Can you work these out from the model? Positions are in its coordinate system, mm. Face numbers are marked on the shaded views. A direction names the side the tool comes from. Give positions to 0.01 mm unless a question says otherwise; leave off trailing zeros. Write each loop counter-clockwise with the first axis right and the second up, starting at its lowest first coordinate (ties: lowest second). Pieces come first, ordered by that corner, then holes.
Autodesk Fusion 360 part; units mm, degrees
sketch "Boceto1" plane through (0, 0, 0) normal (0, 0, 1) x (1, 0, 0)
  line L0 (0, 0) -> (47.682, 0)
  line L1 (47.682, 0) -> (47.682, 36)
  line L2 (47.682, 36) -> (0, 36)
  line L3 (0, 36) -> (0, 0)
  line L4 (4.2944, 26.5117) -> (42.5805, 26.5117)
  line L5 (42.5805, 26.5117) -> (42.5805, 9.2899)
  line L6 (42.5805, 9.2899) -> (4.2944, 9.2899)
  line L7 (4.2944, 9.2899) -> (4.2944, 26.5117)
  circle A0 centre (23.5, 32) radius 2.25
  circle A1 centre (23.5, 4) radius 2.25
  dimension "d8" = 4.5
  dimension "d10" = 4.5
extrude "Extruir1" add sketch "Boceto1" against normal blind 14 contours L0 L1 L2 L3 | L4 L5 L6 L7
sketch "Boceto2" plane through (0, 0, 0) normal (0, 0, 1) x (1, 0, 0)
  circle A0 centre (23.5, 4) radius 2.25
  circle A1 centre (23.5, 32) radius 2.25
  line L0 (0, 36) -> (0, 0)
  line L1 (0, 0) -> (47.682, 0)
  line L2 (47.682, 0) -> (47.682, 36)
  line L3 (47.682, 36) -> (0, 36)
  line L4 (7.6346, 27.7605) -> (39.9467, 27.7605)
  line L5 (39.9467, 27.7605) -> (39.9467, 9.5968)
  line L6 (39.9467, 9.5968) -> (7.6346, 9.5968)
  line L7 (7.6346, 9.5968) -> (7.6346, 27.7605)
extrude "Extruir2" cut sketch "Boceto2" against normal blind 10 contours L4 L5 L6 L7
sketch "Boceto3" plane through (0, 0, -14) normal (0, 0, -1) x (-1, 0, 0)
  circle A0 centre (-23.5, 4) radius 2.25
  circle A1 centre (-23.5, 32) radius 2.25
  line L0 (0, 0) -> (0, 36)
  line L1 (0, 36) -> (-47.682, 36)
  line L2 (-47.682, 36) -> (-47.682, 0)
  line L3 (-47.682, 0) -> (0, 0)
  circle A2 centre (-30, 20) radius 6.5
  circle A3 centre (-15, 20) radius 6.5
  dimension "d25" = 13
  dimension "d26" = 13
extrude "Extruir3" cut sketch "Boceto3" against normal blind 25 contours A2 | A3
thread "Rosca1" thread offset 0 thread length 10
thread "Rosca2" thread offset 0 thread length 10
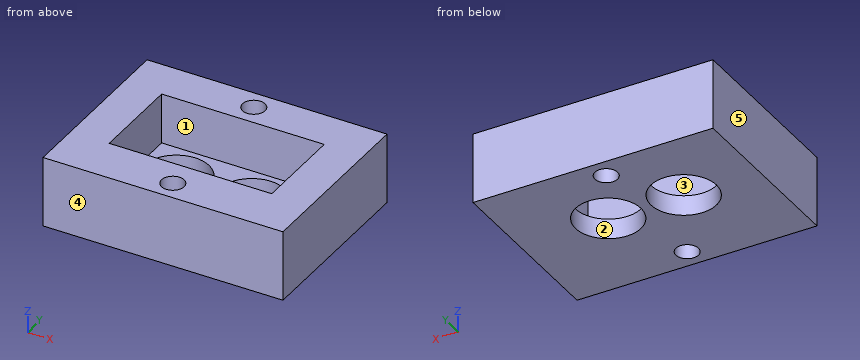
(1) If I drill on L1, parallel to X at y = 20.5, z = -1.75; L2, parallel to Y at x = 17.5, z = -8.75; L3, parallel to X at y = 15.5, z = -12.5, over which ranges is the centre line in solid material (lowest first)?
Returned:
L1: x = 0 to 7.63, 39.95 to 47.68
L2: y = 0 to 9.6, 27.76 to 36
L3: x = 0 to 10.31, 19.69 to 25.31, 34.69 to 47.68
(2) Imagine slicing it at D-D, the plane z = -5.5. Write out the boundary of the cut face in (x, y).
Returned:
outline: (0, 0) - (47.68, 0) - (47.68, 36) - (0, 36) - close; hole (7.63, 9.6) - (39.95, 9.6) - (39.95, 27.76) - (7.63, 27.76) - close; hole circle Ø4.5 at (23.5, 4); hole circle Ø4.5 at (23.5, 32)
(3) For the marked faces 1 and 2, which set-ups out of +Z, -Z, +X, -X, +Y, -Y let a thin tool reach every point of the face, with its end or its side?
Returned:
face 1: +Z
face 2: +Z, -Z
(4) Will this pin go through, and if not, where does the flat tip stop? P1, Ø8, axis at x = 30, y = 20, coming from the -Z side.
Returned:
P1: passes through
(5) Imagine slicing it at B-B, the plane x = 30. Write out the boundary of the cut face in (y, z), plus the area to 3 significant figures.
Returned:
outline: (0, -14) - (13.5, -14) - (13.5, -10) - (9.6, -10) - (9.6, 0) - (0, 0) - close; (26.5, -14) - (36, -14) - (36, 0) - (27.76, 0) - (27.76, -10) - (26.5, -10) - close
area: 270 mm2
(6) If we mould it in two halves opening along Y, with no side actions, what happens to the marked faces 3, 4 and 5? For each: +Y half, -Y half, draft (parallel to the pull), parting line (faces both ways), or undercut.
Returned:
face 3: undercut
face 4: -Y half
face 5: draft
(7) Imagine slicing it at A-A, the plane y = 4. Write out the boundary of the cut face in (x, z).
Returned:
outline: (0, -14) - (21.25, -14) - (21.25, 0) - (0, 0) - close; (25.75, -14) - (47.68, -14) - (47.68, 0) - (25.75, 0) - close
(8) Imagine slicing it at C-C, the plane z = -11.5. Write out the boundary of the cut face in (x, y).
Returned:
outline: (0, 0) - (47.68, 0) - (47.68, 36) - (0, 36) - close; hole circle Ø13 at (15, 20); hole circle Ø4.5 at (23.5, 4); hole circle Ø4.5 at (23.5, 32); hole circle Ø13 at (30, 20)
